from build123d import *

# Parameters (mm, degrees)
SKETCH1_R                                         = 37.846
BOSS_EXTRUDE1_DEPTH                               = 5
SKETCH2_R                                         = 24.846
BOSS_EXTRUDE2_DEPTH                               = 5
SKETCH3_R                                         = 35.56
BOSS_EXTRUDE3_DEPTH                               = 1.6
SKETCH4_R                                         = 2
BOSS_EXTRUDE4_DEPTH                               = 2.5
CIRPATTERN1_COUNT                                 = 3
CSK_FOR_8_FLAT_HEAD_MACHINE_SCREW_100_D           = 4.4958
CSK_FOR_8_FLAT_HEAD_MACHINE_SCREW_100_CSINK_D     = 8.4328
CSK_FOR_8_FLAT_HEAD_MACHINE_SCREW_100_CSINK_ANGLE = 100
BOSS_EXTRUDE5_START                               = -3
SKETCH7_R                                         = 35.56
BOSS_EXTRUDE5_DEPTH                               = 3
CUT_EXTRUDE1_START                                = -1.6
SKETCH8_W                                         = 8
SKETCH8_H                                         = 12
CUT_EXTRUDE1_DEPTH                                = 1.4
CIRPATTERN2_COUNT                                 = 6
SKETCH9_R                                         = 2.2479
CUT_EXTRUDE2_DEPTH                                = 55.208850126


with BuildPart() as part:
    # Sketch1 → Boss-Extrude1 (new body)
    with BuildSketch(Plane(origin=(0, 0, 0), x_dir=(1, 0, 0), z_dir=(0, 1, 0))):
        with Locations(Location((0, 0, 0), (0, 0, 270))):
            Circle(SKETCH1_R)
    extrude(amount=BOSS_EXTRUDE1_DEPTH)

    # Sketch2 → Boss-Extrude2 (add)
    with BuildSketch(Plane(origin=(0, 5, 0), x_dir=(1, 0, 0), z_dir=(0, 1, 0))):
        with Locations(Location((0, 0, 0), (0, 0, 270))):
            Circle(SKETCH2_R)
    extrude(amount=BOSS_EXTRUDE2_DEPTH)

    # Sketch3 → Boss-Extrude3 (add)
    with BuildSketch(Plane(origin=(0, 10, 0), x_dir=(1, 0, 0), z_dir=(0, 1, 0))):
        with Locations(Location((0, 0, 0), (0, 0, 270))):
            Circle(SKETCH3_R)
    extrude(amount=BOSS_EXTRUDE3_DEPTH)

    # Sketch4 → Boss-Extrude4 (add)
    with BuildSketch(Plane(origin=(0, 11.6, 0), x_dir=(1, 0, 0), z_dir=(0, 1, 0))):
        with Locations(Location((0, 10, 0), (0, 0, 270))):
            Circle(SKETCH4_R)
    boss_extrude4 = extrude(amount=BOSS_EXTRUDE4_DEPTH)

    # CirPattern1: Boss-Extrude4 ×3 about axis
    cirpattern1_axis = Axis((0, 0, 0), (0, 1, 0))
    for i in range(1, CIRPATTERN1_COUNT):
        add(boss_extrude4.rotate(cirpattern1_axis, i * 360 / CIRPATTERN1_COUNT))

    # CSK for #8 Flat Head Machine Screw (100)1 (through all)
    with Locations(Plane(origin=(0, 0, 0), x_dir=(-1, 0, 0), z_dir=(0, -1, 0))):
        with Locations((0, 0)):
            CounterSinkHole(CSK_FOR_8_FLAT_HEAD_MACHINE_SCREW_100_D / 2, CSK_FOR_8_FLAT_HEAD_MACHINE_SCREW_100_CSINK_D / 2, counter_sink_angle=CSK_FOR_8_FLAT_HEAD_MACHINE_SCREW_100_CSINK_ANGLE)

    # Sketch7 → Boss-Extrude5 (add)
    with BuildSketch(Plane(origin=(0, 11.6, 0), x_dir=(1, 0, 0), z_dir=(0, 1, 0)).offset(BOSS_EXTRUDE5_START)):
        with Locations(Location((0, 0, 0), (0, 0, 270))):
            Circle(SKETCH7_R)
    extrude(amount=BOSS_EXTRUDE5_DEPTH)

    # Sketch8 → Cut-Extrude1 (cut)
    with BuildSketch(Plane(origin=(0, 11.6, 0), x_dir=(1, 0, 0), z_dir=(0, 1, 0)).offset(CUT_EXTRUDE1_START)):
        with Locations((0, 29.56)):
            Rectangle(SKETCH8_W, SKETCH8_H)
    cut_extrude1 = extrude(amount=-CUT_EXTRUDE1_DEPTH, mode=Mode.SUBTRACT)

    # CirPattern2: Cut-Extrude1 ×6 about axis
    cirpattern2_axis = Axis((0, 0, 0), (0, 1, 0))
    for i in range(1, CIRPATTERN2_COUNT):
        add(cut_extrude1.rotate(cirpattern2_axis, i * 360 / CIRPATTERN2_COUNT), mode=Mode.SUBTRACT)

    # Sketch9 → Cut-Extrude2 (cut, through all)
    with BuildSketch(Plane.XZ.offset(-8.6)):
        with Locations(Location((0, 0, 0), (0, 0, 270))):
            Circle(SKETCH9_R)
    extrude(amount=-CUT_EXTRUDE2_DEPTH, mode=Mode.SUBTRACT)


solid = part.part
For this review, take the finished solid that the model builds, in its own axes (mm). A direction names the side the tool comes from. Give positions to 0.01 mm unless a question says otherwise; leave off trailing zeros. Loops run counter-clockwise (first coordinate to the right, second up) from the corner with the lowest first, then second, coordinate; pieces in that order, holes last.
Item 1: For line 1 along Y through (x, z) = (-31, -2); line 2 along X through (y, z) = (12, 5); line 3 along Y through (x, z) = (28, -19), list the stretches that pass through material, from the lowest coordinate up.
Item 2: Take a section at D-D, the plane z = -28.5. State the section outline as (x, y) points, and give its area (3 significant figures).
Item 3: Draft analysis for pull direction Z (two halves, no side actions). For faces 6 (the cylindrical face through (-1.2, 12.8, -11.6)), 7 (the flat face through (-8, 0, -1)), 8 (the flat face through (21, 8.6, -12)), 9 (the flat face through (-21, 8.6, 12)), state which applies: +Z half, -Z half, draft (parallel to the pull), parting line (faces both ways), or undercut.
Item 4: Tool access review of faces 1 (the cylindrical face through (-21.638, 10.079, -28.219)), 2 (the flat face through (-23.431, 9.31, 18.146)), 3 (the flat face through (16, 8.6, 25)), 4 (the flat face through (23.431, 9.31, 18.146)), 5 (the flat face through (-20.432, 9.31, -11.732)): name each direction out of +Z, -Z, +X, -X, +Y, -Y from which nothing blocks a thin tool from reaching the whole face with its end or side.
Item 5: Take a section at C-C, the plane y = 3.25. State the section outline as (x, z) points, and give its area (3 significant figures).
Item 6: Take a section at B-B, the plane z = 0. State the section outline as (x, y) points, and give its area (3 significant figures).
Item 7: Take a section at A-A, the plane x = 0. State the section outline as (y, z) points.
Item 8: Insertion check: pin 1 (4 mm diameter, centred on x = 28, y = 10.5, fed in from -Z); pin 2 (1.4 mm diameter, centred on x = -19.5, z = 10.5, fed in from +Y); pin 3 (1.5 mm diameter, centred on y = 5, z = -22.5, fed in from +X). Each pin has a flat end and moves straight along its axis. Give the tip position at first contact, or say it passes through.
Calculated:
1. line 1: y = 0 to 5, 8.6 to 11.6
1. line 2: x = -10.66 to -6.66, 6.66 to 10.66
1. line 3: y = 0 to 5, 10 to 11.6
2. outline: (-24.9, 0) - (24.9, 0) - (24.9, 5) - (-24.9, 5) - close; (-21.27, 8.6) - (-4, 8.6) - (-4, 10) - (4, 10) - (4, 8.6) - (21.27, 8.6) - (21.27, 11.6) - (-21.27, 11.6) - close
2. area: 365 mm2
3. face 6: parting line
3. face 7: draft
3. face 8: undercut
3. face 9: undercut
4. face 1: +Y
4. face 2: -X
4. face 3: +Z, +X
4. face 4: +X
4. face 5: none
5. outline: circle Ø75.69 at (0, 0); hole circle Ø4.5 at (0, 0)
5. area: 4,480 mm2
6. outline: (-37.85, 0) - (-4.22, 0) - (-2.25, 1.65) - (-2.25, 11.6) - (-35.56, 11.6) - (-35.56, 8.6) - (-24.85, 8.6) - (-24.85, 5) - (-37.85, 5) - close; (2.25, 1.65) - (4.22, 0) - (37.85, 0) - (37.85, 5) - (24.85, 5) - (24.85, 8.6) - (35.56, 8.6) - (35.56, 11.6) - (2.25, 11.6) - close
6. area: 715 mm2
7. outline: (0, -37.85) - (5, -37.85) - (5, -24.85) - (8.6, -24.85) - (8.6, -23.56) - (10, -23.56) - (10, -35.56) - (11.6, -35.56) - (11.6, -12) - (14.1, -12) - (14.1, -8) - (11.6, -8) - (11.6, -2.25) - (1.65, -2.25) - (0, -4.22) - close; (0, 4.22) - (1.65, 2.25) - (11.6, 2.25) - (11.6, 35.56) - (10, 35.56) - (10, 23.56) - (8.6, 23.56) - (8.6, 24.85) - (5, 24.85) - (5, 37.85) - (0, 37.85) - close
8. pin 1: stops at z = -24.26
8. pin 2: stops at y = 11.6
8. pin 3: stops at x = 30.97
